```python
from build123d import *
from build123d.topology import SkipClean

# Parameters (mm, degrees)
SKETCH_1_R                 = 0.5
SKETCH_1_R_2               = 6.5
EXTRUDE_2_DEPTH            = 2
HOLE_WIZARD_M31_AT_2_COUNT = 2
HOLE_WIZARD_M31_AT_2_PITCH = 10.338881425
HOLE_WIZARD_M31_AT_3_COUNT = 2
HOLE_WIZARD_M31_AT_3_PITCH = 20.124611797
HOLE_WIZARD_M31_AT_4_COUNT = 2
HOLE_WIZARD_M31_AT_4_PITCH = 45
HOLE_WIZARD_M31_AT_5_COUNT = 2
HOLE_WIZARD_M31_AT_5_PITCH = 43.796204526
HOLE_WIZARD_M31_AT_6_COUNT = 2
HOLE_WIZARD_M31_AT_6_PITCH = 45.190407637
EXTRUDE_START              = 0.5
SKETCH_4_R                 = 8.5
SKETCH_4_R_2               = 6.5
EXTRUDE_3_DEPTH            = 0.5
EXTRUDE_START_2            = 5.1
SKETCH_5_R                 = 7.5
SKETCH_5_R_2               = 6.5
EXTRUDE_4_DEPTH            = 5.1
CUT_EXTRUDE_1_DEPTH        = 1
EXTRUDE_START_3            = 1
EXTRUDE_5_DEPTH            = 1


with BuildPart() as part:
    # Эскиз1 → Бобышка-Вытянуть2 (new body)
    with BuildSketch(Plane.XY):
        with BuildLine():
            Line((-5.16821295, 17.764543293), (-21.057898637, 13.951904294))
            ThreePointArc((-21.057898637, 13.951904294), (-22.612693727, 13.19430978), (-23.702320561, 11.851160281))
            ThreePointArc((-23.702320561, 11.851160281), (-26.5, 0), (-23.702320561, -11.851160281))
            ThreePointArc((-23.702320561, -11.851160281), (-22.612693727, -13.19430978), (-21.057898637, -13.951904294))
            Line((-21.057898637, -13.951904294), (-5.16821295, -17.764543293))
            ThreePointArc((-5.16821295, -17.764543293), (0, -18.50106547), (5.16821295, -17.764543293))
            Line((5.16821295, -17.764543293), (21.057898637, -13.951904294))
            ThreePointArc((21.057898637, -13.951904294), (22.612693727, -13.19430978), (23.702320561, -11.851160281))
            ThreePointArc((23.702320561, -11.851160281), (25.169556704, -8.291164895), (26.105397143, -4.556121157))
            Line((26.105397143, -4.556121157), (29.049405058, 12.312283599))
            ThreePointArc((29.049405058, 12.312283599), (28.170900607, 15.573823459), (25.108967753, 17))
            Line((25.108967753, 17), (7.299960514, 17))
            ThreePointArc((7.299960514, 17), (1.132350887, 18.466380397), (-5.16821295, 17.764543293))
        make_face()
        with Locations((25, 12.5)):
            Circle(SKETCH_1_R, mode=Mode.SUBTRACT)
        with Locations((22.5, 0)):
            Circle(SKETCH_1_R, mode=Mode.SUBTRACT)
        with Locations((20.124611797, -10.062305899)):
            Circle(SKETCH_1_R, mode=Mode.SUBTRACT)
        with Locations(Location((-20.124611797, -10.062305899, 0), (0, 0, 180))):
            Circle(SKETCH_1_R, mode=Mode.SUBTRACT)
        with Locations(Location((-22.5, 0, 0), (0, 0, 180))):
            Circle(SKETCH_1_R, mode=Mode.SUBTRACT)
        with Locations((-20.124611797, 10.062305899)):
            Circle(SKETCH_1_R, mode=Mode.SUBTRACT)
        Circle(SKETCH_1_R_2, mode=Mode.SUBTRACT)
    extrude(amount=EXTRUDE_2_DEPTH)

    # Эскиз3 → Зенковка для винта с потайной головкой и внутренним шестигранником M31 (revolve, cut)
    with BuildSketch(Plane(origin=(-20.124611797, 10.062305899, 2), x_dir=(0, -1, 0), z_dir=(1, 0, 0))):
        Polygon((0, 0), (0, 2), (1.7, 2), (1.7, 1.66), (3.36, 0), align=None)
    hole_wizard_m31 = revolve(axis=Axis((-20.124611797, 10.062305899, 8.35), (0, 0, -1)), mode=Mode.SUBTRACT)

    # Зенковка для винта с потайной головкой и внутренним шестигранником M31 at 2: Зенковка для винта с потайной головкой и внутренним шестигранником M31 ×2
    with Locations(*[Vector(-0.2297529205473615, -0.9732489894677301, 0) * (i * HOLE_WIZARD_M31_AT_2_PITCH) for i in range(1, HOLE_WIZARD_M31_AT_2_COUNT)]):
        add(hole_wizard_m31, mode=Mode.SUBTRACT)

    # Зенковка для винта с потайной головкой и внутренним шестигранником M31 at 3: Зенковка для винта с потайной головкой и внутренним шестигранником M31 ×2
    with Locations(*[(0, -i * HOLE_WIZARD_M31_AT_3_PITCH, 0) for i in range(1, HOLE_WIZARD_M31_AT_3_COUNT)]):
        add(hole_wizard_m31, mode=Mode.SUBTRACT)

    # Зенковка для винта с потайной головкой и внутренним шестигранником M31 at 4: Зенковка для винта с потайной головкой и внутренним шестигранником M31 ×2
    with Locations(*[Vector(0.894427190999916, -0.4472135954999578, 0) * (i * HOLE_WIZARD_M31_AT_4_PITCH) for i in range(1, HOLE_WIZARD_M31_AT_4_COUNT)]):
        add(hole_wizard_m31, mode=Mode.SUBTRACT)

    # Зенковка для винта с потайной головкой и внутренним шестигранником M31 at 5: Зенковка для винта с потайной головкой и внутренним шестигранником M31 ×2
    with Locations(*[Vector(0.9732489894677302, -0.2297529205473611, 0) * (i * HOLE_WIZARD_M31_AT_5_PITCH) for i in range(1, HOLE_WIZARD_M31_AT_5_COUNT)]):
        add(hole_wizard_m31, mode=Mode.SUBTRACT)

    # Зенковка для винта с потайной головкой и внутренним шестигранником M31 at 6: Зенковка для винта с потайной головкой и внутренним шестигранником M31 ×2
    with Locations(*[Vector(0.9985440308456991, 0.0539427331753181, 0) * (i * HOLE_WIZARD_M31_AT_6_PITCH) for i in range(1, HOLE_WIZARD_M31_AT_6_COUNT)]):
        add(hole_wizard_m31, mode=Mode.SUBTRACT)

    # Эскиз4 → Бобышка-Вытянуть3 (add)
    with SkipClean():  # the faces are left unmerged after this step: merging them gives an invalid solid
        with BuildSketch(Plane(origin=(0, 0, 0), x_dir=(-1, 0, 0), z_dir=(0, 0, -1)).offset(EXTRUDE_START)):
            with Locations(Location((0, 0, 0), (0, 0, 180))):
                Circle(SKETCH_4_R)
            Circle(SKETCH_4_R_2, mode=Mode.SUBTRACT)
        extrude(amount=-EXTRUDE_3_DEPTH)

    # Эскиз5 → Бобышка-Вытянуть4 (add)
    with SkipClean():  # the faces are left unmerged after this step: merging them gives an invalid solid
        with BuildSketch(Plane(origin=(0, 0, -0.5), x_dir=(-1, 0, 0), z_dir=(0, 0, -1)).offset(EXTRUDE_START_2)):
            Circle(SKETCH_5_R)
            Circle(SKETCH_5_R_2, mode=Mode.SUBTRACT)
        extrude(amount=-EXTRUDE_4_DEPTH)

    # Эскиз6 → Вырез-Вытянуть1 (cut)
    with SkipClean():  # the faces are left unmerged after this step: merging them gives an invalid solid
        with BuildSketch(Plane.XY.offset(2)):
            with BuildLine():
                Line((-5.119475911, 4.77398852), (15.340474891, 26.714599569))
                Line((15.340474891, 26.714599569), (25.579426713, 17.166622528))
                Line((25.579426713, 17.166622528), (5.119475911, -4.77398852))
                ThreePointArc((5.119475911, -4.77398852), (-4.77398852, -5.119475911), (-5.119475911, 4.77398852))
            make_face()
        extrude(amount=-CUT_EXTRUDE_1_DEPTH, mode=Mode.SUBTRACT)

    # Эскиз7 → Бобышка-Вытянуть5 (add)
    with SkipClean():  # the faces are left unmerged after this step: merging them gives an invalid solid
        with BuildSketch(Plane(origin=(0, 0, -5.6), x_dir=(-1, 0, 0), z_dir=(0, 0, -1)).offset(EXTRUDE_START_3)):
            with BuildLine():
                Line((-1.941142838, 7.244443697), (-1.682323793, 6.278517871))
                ThreePointArc((-1.682323793, 6.278517871), (0, 6.5), (1.682323793, 6.278517871))
                Line((1.682323793, 6.278517871), (1.941142838, 7.244443697))
                ThreePointArc((1.941142838, 7.244443697), (0, 7.5), (-1.941142838, 7.244443697))
            make_face()
            with BuildLine():
                Line((5.303300859, 5.303300859), (4.596194078, 4.596194078))
                ThreePointArc((4.596194078, 4.596194078), (5.629165125, 3.25), (6.278517871, 1.682323793))
                Line((6.278517871, 1.682323793), (7.244443697, 1.941142838))
                ThreePointArc((7.244443697, 1.941142838), (6.495190528, 3.75), (5.303300859, 5.303300859))
            make_face()
            with BuildLine():
                Line((7.244443697, -1.941142838), (6.278517871, -1.682323793))
                ThreePointArc((6.278517871, -1.682323793), (5.629165125, -3.25), (4.596194078, -4.596194078))
                Line((4.596194078, -4.596194078), (5.303300859, -5.303300859))
                ThreePointArc((5.303300859, -5.303300859), (6.495190528, -3.75), (7.244443697, -1.941142838))
            make_face()
            with BuildLine():
                Line((1.941142838, -7.244443697), (1.682323793, -6.278517871))
                ThreePointArc((1.682323793, -6.278517871), (0, -6.5), (-1.682323793, -6.278517871))
                Line((-1.682323793, -6.278517871), (-1.941142838, -7.244443697))
                ThreePointArc((-1.941142838, -7.244443697), (0, -7.5), (1.941142838, -7.244443697))
            make_face()
            with BuildLine():
                Line((-5.303300859, -5.303300859), (-4.596194078, -4.596194078))
                ThreePointArc((-4.596194078, -4.596194078), (-5.629165125, -3.25), (-6.278517871, -1.682323793))
                Line((-6.278517871, -1.682323793), (-7.244443697, -1.941142838))
                ThreePointArc((-7.244443697, -1.941142838), (-6.495190528, -3.75), (-5.303300859, -5.303300859))
            make_face()
            with BuildLine():
                Line((-7.244443697, 1.941142838), (-6.278517871, 1.682323793))
                ThreePointArc((-6.278517871, 1.682323793), (-5.629165125, 3.25), (-4.596194078, 4.596194078))
                Line((-4.596194078, 4.596194078), (-5.303300859, 5.303300859))
                ThreePointArc((-5.303300859, 5.303300859), (-6.495190528, 3.75), (-7.244443697, 1.941142838))
            make_face()
        extrude(amount=-EXTRUDE_5_DEPTH)


solid = part.part
```
Here's how the part is built. I have some questions about the finished solid (model axes, mm). A direction names the side the tool comes from. Give positions to 0.01 mm unless a question says otherwise; leave off trailing zeros. Order: outer loops, then holes, each group sorted by start corner. A loop starts at its lowest first (then second) coordinate and runs counter-clockwise, first axis right, second up. Notation, with made-up numbers: M 14,44.25 L 56,44.25 A35 cw 56,82.25 Z; hole C -33.75,77 d8. An arc over 180 degrees is marked long. Use a Markdown table: item, result. Add a question column.
1. Suppose I cut it at D-D (x = 14.5). List the corners of the cut face in (y, z) for me, and give its area (3 significant figures).
2. Suppose I cut it at C-C (z = -2.5). List the corners of the cut face in (x, y) for me, and give its area (3 significant figures).
3. Suppose I cut it at B-B (x = -3). List the corners of the cut face in (y, z) for me.
4. On a 3-axis mill with a long thin cutter (end or side, diameter ignored), from which of +Z, -Z, +X, -X, +Y, -Y can I reach the whole of each face in a straight line? I mean faces 5 (the flat face through (0.64, 10.95, 1.51)), 6 (the flat face through (7, 8, 0)), 7 (the cylindrical face through (-20.635, 8.441, 0.172)). Say none if no direction works.
5. I need wall thicknesses on probe 1 along Y at (x, z) = (0, 0.45); probe 2 along Y at (x, z) = (0, -0.2); probe 3 along Z at (x, y) = (11, -9). Which ranges of each line are inside material? Lowest first, please. Write a range as from..to.
6. For pin 1 Ø2 at (y, z) = (3, -4) entering from +X; pin 2 Ø5 at (y, z) = (13, -2) entering from -X; pin 3 Ø1 at (y, z) = (-2.5, -2) entering from -X; pin 4 Ø2.5 at (x, y) = (22.5, 0) entering from +Z (3 decimals), each with a flat end and sliding along its axis, tell me the tip position at first contact or that it passes through.
7. Suppose I cut it at A-A (y = 0). Give the number of separate pieces and of enclosed holes in the cut face, and give its area (3 significant figures).
8. If we mould it in two halves opening along Y, with no side actions, what happens to faces 1 (the flat face through (0, 8, -0.5)), 2 (the cylindrical face through (24.16, 0.37, 0.17)), 3 (the flat face through (-13.002, 15.885, 0.986)), 4 (the flat face through (10, 9, 1))? For each: +Y half, -Y half, draft (parallel to the pull), parting line (faces both ways), or undercut.
Results list:
| question | item | result |
|---|---|---|
| 1 | outline | M -15.53,0 L 17,0 L 17,1 L 5.29,1 L 5.29,2 L -15.53,2 Z |
| 1 | area | 53.3 mm² |
| 2 | outline | C 0,0 d15; hole C 0,0 d13 |
| 2 | area | 44.0 mm² |
| 3 | outline | M -18.26,0 L -7.95,0 L -7.95,-0.5 L -6.87,-0.5 L -6.87,-5.6 L -5.77,-5.6 L -5.77,1 L -6.32,1 L -6.32,2 L -18.26,2 Z; M 5.77,-5.6 L 6.87,-5.6 L 6.87,-0.5 L 7.95,-0.5 L 7.95,0 L 18.26,0 L 18.26,2 L 7.05,2 L 7.05,1 L 5.77,1 Z |
| 4 | face 5 | +Z |
| 4 | face 6 | -Z |
| 4 | face 7 | +Z, -Z |
| 5 | probe 1 | y = -18.5..-6.5, 6.5..18.5 |
| 5 | probe 2 | y = -8.5..-6.5, 6.5..8.5 |
| 5 | probe 3 | z = 0..2 |
| 6 | pin 1 | stops at x = 7.23 |
| 6 | pin 2 | stops at x = -23.87 |
| 6 | pin 3 | stops at x = -7.23 |
| 6 | pin 4 | passes through |
| 7 | separate pieces | 4 |
| 7 | enclosed holes | 0 |
| 7 | area | 70.3 mm² |
| 8 | face 1 | draft |
| 8 | face 2 | undercut |
| 8 | face 3 | +Y half |
| 8 | face 4 | undercut |
